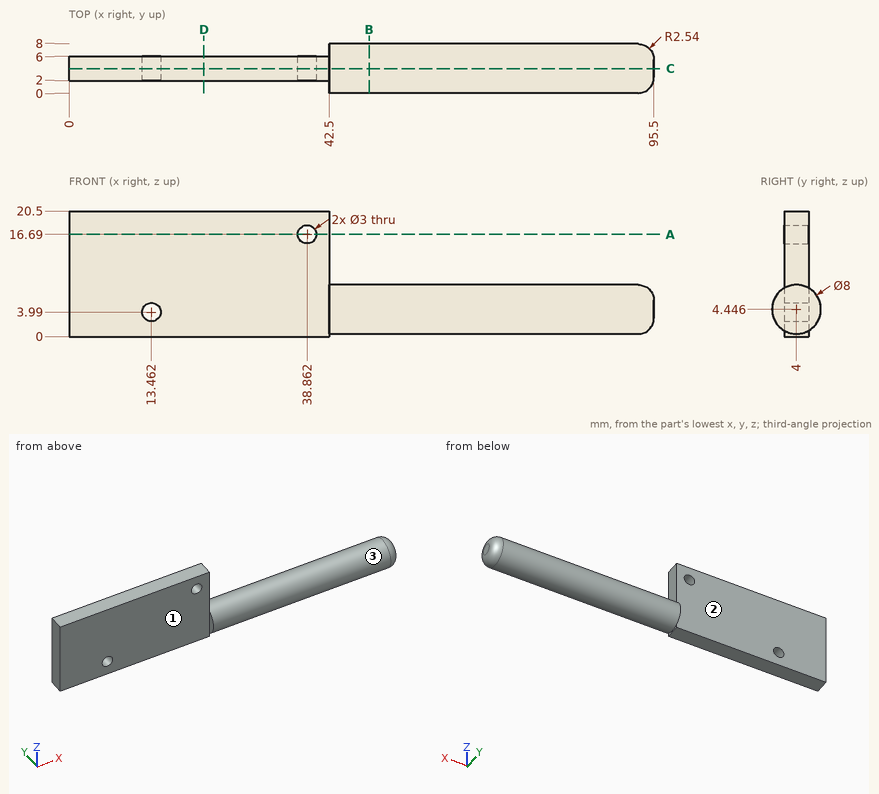
Source: three-view drawing plus pictorial views. Frame: mm from the lowest corner of the part. A direction names the side the tool comes from. Give positions to 0.01 mm unless a question says otherwise; leave off trailing zeros. Loops run counter-clockwise (first coordinate to the right, second up) from the corner with the lowest first, then second, coordinate; pieces in that order, holes last.
1) Section query D-D on x = 22. Return the cut outline in (y, z), and give its area (3 significant figures).
A:
outline: (2, 0) - (6, 0) - (6, 20.5) - (2, 20.5) - close
area: 82.0 mm2
2) Line query: L1, parallel to X at y = 3.85, z = 3.99; L2, parallel to X at y = 4.5, z = 16.75; L3, parallel to Z at x = 63.5, y = 2. Output: solid intervals per line, ascending.
A:
L1: x = 0 to 11.96, 14.96 to 95.5
L2: x = 0 to 37.36, 40.36 to 42.5
L3: z = 0.98 to 7.91
3) Section query C-C on y = 4. Count the separate pieces of the cut face and the enclosed holes in it, and give its area (3 significant figures).
A:
separate pieces: 1
enclosed holes: 2
area: 1,280 mm2
4) Section query A-A on z = 16.69. Return the cut outline in (x, y), and give its area (3 significant figures).
A:
outline: (0, 2) - (37.36, 2) - (37.36, 6) - (0, 6) - close; (40.36, 2) - (42.5, 2) - (42.5, 6) - (40.36, 6) - close
area: 158 mm2
5) Section query B-B on x = 49. Return the cut outline in (y, z) (1 decimal).
A:
outline: circle Ø8 at (4, 4.4)
6) Reachability of the marked faces 1, 2 and 3 from +Z, -Z, +X, -X, +Y, -Y: full face, straight path, thin tool, end or side. Return the list, or none.
A:
face 1: +Z, -Z, -X, -Y
face 2: +Z, -Z, -X, +Y
face 3: +X
7) Contact query for flat-ended pins moving along their axis: pin 1 (4 mm diameter, centred on x = 38.862, z = 16.69, fed in from +Y); pin 2 (2.5 mm diameter, centred on x = 13.462, z = 3.99, fed in from +Y); pin 3 (0.6 mm diameter, centred on y = 7, z = 3, fed in from -X); pin 4 (1.2 mm diameter, centred on y = 4, z = 16, fed in from +X). Output: stop coordinate, or through.
A:
pin 1: stops at y = 6
pin 2: passes through
pin 3: stops at x = 42.5
pin 4: stops at x = 42.5
